```python
from build123d import *

# Parameters (mm, degrees)
EXTRUDE_1_DEPTH          = 96.5
CHAMFER_1_SIZE           = 1
CHAMFER_2_SIZE           = 1
CUT_EXTRUDE_1_DEPTH      = 98.010617976
CUT_EXTRUDE_1_DEPTH_BACK = 10
SKETCH_2_R               = 1.2
SKETCH_2_3_R             = 2.05
CUT_EXTRUDE_2_DEPTH      = 2
CHAMFER_3_SIZE           = 2
SKETCH_3_W               = 1.8
SKETCH_3_H               = 7.4
CUT_EXTRUDE_3_DEPTH      = 1.9
CHAMFER_4_SIZE           = 0.2
CHAMFER_5_SIZE           = 0.6


with BuildPart() as part:
    # 草图1 → 凸台-拉伸1 (new body)
    with BuildSketch(Plane.XY):
        Polygon((0, 0), (8, 0), (8, 4), (0, 4), (-1.8, 4), (-1.8, -1.9), (0, -1.9), align=None)
    extrude(amount=-EXTRUDE_1_DEPTH)

    # 倒角1
    chamfer_1_edges = [part.edges().sort_by_distance(p)[0] for p in [
        (8, 0, -48.25),
    ]]
    chamfer(chamfer_1_edges, length=CHAMFER_1_SIZE)

    # 倒角2
    chamfer_2_edges = [part.edges().sort_by_distance(p)[0] for p in [
        (8, 4, -48.25),
    ]]
    chamfer(chamfer_2_edges, length=CHAMFER_2_SIZE)

    # 草图2 → 切除-拉伸1 (cut, two sides: drawn at the far end of the back side and taken through both)
    with BuildSketch(Plane(origin=(0, 4, 0), x_dir=(1, 0, 0), z_dir=(0, 1, 0)).offset(-CUT_EXTRUDE_1_DEPTH_BACK)):
        with Locations(Location((5.2, 79.25, 0), (0, 0, 90))):
            Circle(SKETCH_2_R)
        with Locations(Location((5.2, 17.25, 0), (0, 0, 90))):
            Circle(SKETCH_2_R)
    extrude(amount=CUT_EXTRUDE_1_DEPTH + CUT_EXTRUDE_1_DEPTH_BACK, mode=Mode.SUBTRACT)

    # 草图2<3> → 切除-拉伸2 (cut)
    with BuildSketch(Plane(origin=(0, 4, 0), x_dir=(1, 0, 0), z_dir=(0, 1, 0))):
        with Locations(Location((5.2, 79.25, 0), (0, 0, 270))):
            Circle(SKETCH_2_3_R)
        with Locations(Location((5.2, 17.25, 0), (0, 0, 270))):
            Circle(SKETCH_2_3_R)
    extrude(amount=-CUT_EXTRUDE_2_DEPTH, mode=Mode.SUBTRACT)

    # 倒角3
    chamfer_3_edges = [part.edges().sort_by_distance(p)[0] for p in [
        (-1.8, 4, -48.25),
    ]]
    chamfer(chamfer_3_edges, length=CHAMFER_3_SIZE)

    # 草图3 → 切除-拉伸3 (cut)
    with BuildSketch(Plane.XZ.offset(1.9)):
        with Locations((-0.9, -92.8)):
            Rectangle(SKETCH_3_W, SKETCH_3_H)
        with Locations((-0.9, -3.7)):
            Rectangle(SKETCH_3_W, SKETCH_3_H)
    extrude(amount=-CUT_EXTRUDE_3_DEPTH, mode=Mode.SUBTRACT)

    # 倒角4
    chamfer_4_edges = [part.edges().sort_by_distance(p)[0] for p in [
        (-1.8, -1.9, -48.25),
        (0, -1.9, -48.25),
        (-1.8, -0.95, -89.1),
        (0, -0.95, -89.1),
        (-1.8, 0, -92.8),
        (-1.8, -0.95, -7.4),
        (0, -0.95, -7.4),
        (-1.8, 0, -3.7),
    ]]
    chamfer(chamfer_4_edges, length=CHAMFER_4_SIZE)

    # 倒角5
    # the kernel refuses this chamfer: 0.6 mm, written as the material it takes off along each edge
    with BuildSketch(Plane(origin=(1.343009793, -1.9, -89.1), x_dir=(0, 0.9996219169112965, -0.027495876610595982), z_dir=(-1, 0, 0))) as chamfer_5_piece_1:
        Polygon((CHAMFER_5_SIZE * 0.999621916911, -CHAMFER_5_SIZE * 0.0274958766106), (-CHAMFER_5_SIZE * 0.0274958766106, -CHAMFER_5_SIZE * 0.999621916911), (0, 0), align=None)
    extrude(amount=4.486019586, mode=Mode.SUBTRACT)
    with BuildSketch(Plane(origin=(1.343009793, -1.9, -7.4), x_dir=(0, 0.9996219169112968, 0.027495876610585925), z_dir=(-1, 0, 0))) as chamfer_5_piece_2:
        Polygon((CHAMFER_5_SIZE * 0.999621916911, CHAMFER_5_SIZE * 0.0274958766106), (-CHAMFER_5_SIZE * 0.0274958766106, CHAMFER_5_SIZE * 0.999621916911), (0, 0), align=None)
    extrude(amount=4.486019586, mode=Mode.SUBTRACT)


solid = part.part
```
Source: CAD feature listing. Evaluate the final solid. Frame: model axes, mm. A direction names the side the tool comes from. Coordinates: 2 decimals unless noted, no trailing zeros. Loops run counter-clockwise (first coordinate to the right, second up) from the corner with the lowest first, then second, coordinate; pieces in that order, holes last. Notation, with made-up numbers: (51.25, -35) -> (105.25, -35) arc R8 ccw to (105.25, -25) -> close; hole circle Ø3 at (-7, 33.5). An arc over 180 degrees is marked (long way). One line per item, written item: value. Start each with the question number.
Q1. Contact query for flat-ended pins moving along their axis: P1, Ø1.4, axis at x = -1, y = -1, coming from the +Z side; P2, Ø1.2, axis at x = 4.5, z = -79.5, coming from the +Y side; P3, Ø1, axis at x = -0.5, y = -1, coming from the -Z side. Output: stop coordinate, or through.
Q2. Set-up query: faces 1 (the face through (0, -1, -48)), 2 (the face through (5.66, 0.99, -80.36)), 3 (the face through (4, 2, -16)). Return all of +Z, -Z, +X, -X, +Y, -Y with unobstructed straight access to the full face (end or side cutting, diameter ignored); none if empty.
Q3. Section query C-C, the plane z = -33.5. Return the cut outline in (x, y), and give its area (3 significant figures).
Q4. Line query: line 1 along Z through (x, y) = (5.2, 3.1); line 2 along X through (y, z) = (1.2, -79.25); line 3 along Y through (x, z) = (5.5, -35). Output: solid intervals per line, ascending.
Q5. Mould query, pull axis Z, two halves, no side actions, for faces 4 (the face through (4, 2, -78)), 5 (the face through (5.93, 0.99, -16.3)), 6 (the face through (8, 2, -48)), 7 (the face through (3, 2, -96.5)). Classes: pulls with the +Z half, pulls with the -Z half, needs draft (parallel to the pull), parting line crosses it, or undercut.
Q6. Section query B-B, the plane x = 5.2. Return the cut outline in (y, z), and give its area (3 significant figures).
Q7. Section query A-A, the plane z = -79.25. Return the cut outline in (x, y), and give its area (3 significant figures).
Results:
1. P1: z = -7.4
1. P2: y = 2
1. P3: z = -89.1
2. face 1: +Z, -Z, +X, -Y
2. face 2: +Y, -Y
2. face 3: +Y
3. outline: (-1.8, -1.7) -> (-1.6, -1.9) -> (-0.2, -1.9) -> (0, -1.7) -> (0, 0) -> (7, 0) -> (8, 1) -> (8, 3) -> (7, 4) -> (0.2, 4) -> (-1.8, 2) -> close
3. area: 39.6 mm^2
4. line 1: -96.5 to -81.3, -77.2 to -19.3, -15.2 to 0
4. line 2: -1.8 to 4, 6.4 to 8
4. line 3: 0 to 4
5. face 4: undercut
5. face 5: undercut
5. face 6: needs draft
5. face 7: pulls with the -Z half
6. outline: (0, -96.5) -> (4, -96.5) -> (4, -81.3) -> (2, -81.3) -> (2, -80.45) -> (0, -80.45) -> close; (0, -78.05) -> (2, -78.05) -> (2, -77.2) -> (4, -77.2) -> (4, -19.3) -> (2, -19.3) -> (2, -18.45) -> (0, -18.45) -> close; (0, -16.05) -> (2, -16.05) -> (2, -15.2) -> (4, -15.2) -> (4, 0) -> (0, 0) -> close
6. area: 360 mm^2
7. outline: (-1.8, -1.7) -> (-1.6, -1.9) -> (-0.2, -1.9) -> (0, -1.7) -> (0, 0) -> (4, 0) -> (4, 2) -> (3.15, 2) -> (3.15, 4) -> (0.2, 4) -> (-1.8, 2) -> close; (6.4, 0) -> (7, 0) -> (8, 1) -> (8, 3) -> (7.25, 3.75) -> (7.25, 2) -> (6.4, 2) -> close
7. area: 26.6 mm^2
